```python
from build123d import *

# Parameters (mm, degrees)
BODY_DEPTH               = 10
SKETCH2_R                = 7.25
SPRING_HOLE_DEPTH        = 10
SKETCH3_R                = 3.25
SHAFT_HOLE_DEPTH         = 51.249378106
FIXATION_HOLE_START      = -20
SKETCH4_R                = 2.75
FIXATION_HOLE_DEPTH      = 72.478150705
SKETCH6_W                = 6
SKETCH6_H                = 10.5
NUT_HOLE_DEPTH           = 20
SKETCH7_R                = 3.2
INSERTS_TOP_DEPTH        = 9.5
SKETCH8_R                = 4.5
M5_SCREW_PLACE_DEPTH     = 5
SKETCH9_R                = 6.2
LINEARBEARINGPLACE_DEPTH = 19
CHAMFER1_SIZE            = 1
CHAMFER2_SIZE            = 1


with BuildPart() as part:
    # Sketch1 → Body (new, symmetric)
    with BuildSketch(Plane(origin=(0, 0, 0), x_dir=(1, 0, 0), z_dir=(0, 1, 0))):
        Polygon((-45, 15), (45, 15), (45, -5), (45, -15), (25, -15), (25, 0), (-25, 0), (-25, -15), (-45, -15), (-45, -5), align=None)
    extrude(amount=BODY_DEPTH, both=True)

    # Sketch2 → Spring_Hole (cut)
    with BuildSketch(Plane.XY.offset(15)):
        with Locations((-35, 0)):
            Circle(SKETCH2_R)
    spring_hole = extrude(amount=-SPRING_HOLE_DEPTH, mode=Mode.SUBTRACT)

    # Sketch3 → Shaft_Hole (cut, symmetric)
    with BuildSketch(Plane.XY.offset(5)):
        with Locations((-35, 0)):
            Circle(SKETCH3_R)
    shaft_hole = extrude(amount=SHAFT_HOLE_DEPTH, both=True, mode=Mode.SUBTRACT)

    # Sketch4 → Fixation_Hole (cut, through all)
    with BuildSketch(Plane(origin=(0, 10, 0), x_dir=(1, 0, 0), z_dir=(0, 1, 0)).offset(FIXATION_HOLE_START)):
        with Locations(Location((-18, 7.5, 0), (0, 0, 270))):
            Circle(SKETCH4_R)
    fixation_hole = extrude(amount=FIXATION_HOLE_DEPTH, mode=Mode.SUBTRACT)

    # Sketch6 → Nut_Hole (cut)
    with BuildSketch(Plane.ZY.offset(45)):
        with Locations((-7.5, 0)):
            Rectangle(SKETCH6_W, SKETCH6_H)
    nut_hole = extrude(amount=-NUT_HOLE_DEPTH, mode=Mode.SUBTRACT)

    # Mirror1: Spring_Hole, Shaft_Hole, Fixation_Hole, Nut_Hole across plane
    add(spring_hole.mirror(Plane(origin=(0, 0, 0), x_dir=(0, 0, 1), z_dir=(1, 0, 0))), mode=Mode.SUBTRACT)
    add(shaft_hole.mirror(Plane(origin=(0, 0, 0), x_dir=(0, 0, 1), z_dir=(1, 0, 0))), mode=Mode.SUBTRACT)
    add(fixation_hole.mirror(Plane(origin=(0, 0, 0), x_dir=(0, 0, 1), z_dir=(1, 0, 0))), mode=Mode.SUBTRACT)
    add(nut_hole.mirror(Plane(origin=(0, 0, 0), x_dir=(0, 0, 1), z_dir=(1, 0, 0))), mode=Mode.SUBTRACT)

    # Sketch7 → Inserts_Top (cut)
    with BuildSketch(Plane(origin=(0, 0, -15), x_dir=(-1, 0, 0), z_dir=(0, 0, -1))):
        with Locations((-10, 0)):
            Circle(SKETCH7_R)
        with Locations(Location((10, 0, 0), (0, 0, 180))):
            Circle(SKETCH7_R)
    extrude(amount=-INSERTS_TOP_DEPTH, mode=Mode.SUBTRACT)

    # Sketch8 → M5_Screw_Place (cut)
    with BuildSketch(Plane.XZ.offset(10)):
        with Locations(Location((-18, -7.5, 0), (0, 0, 270))):
            Circle(SKETCH8_R)
        with Locations(Location((18, -7.5, 0), (0, 0, 270))):
            Circle(SKETCH8_R)
    extrude(amount=-M5_SCREW_PLACE_DEPTH, mode=Mode.SUBTRACT)

    # Sketch9 → LinearBearingPlace (cut)
    with BuildSketch(Plane(origin=(0, 0, -15), x_dir=(-1, 0, 0), z_dir=(0, 0, -1))):
        with Locations((-35, 0)):
            Circle(SKETCH9_R)
    linearbearingplace = extrude(amount=-LINEARBEARINGPLACE_DEPTH, mode=Mode.SUBTRACT)

    # Mirror2: LinearBearingPlace across plane
    add(linearbearingplace.mirror(Plane(origin=(0, 0, 0), x_dir=(0, 0, 1), z_dir=(1, 0, 0))), mode=Mode.SUBTRACT)

    # Chamfer1
    chamfer1_edges = [part.edges().sort_by_distance(p)[0] for p in [
        (0, -10, 0),
        (-25, -10, 7.5),
        (-35, -10, 15),
        (-45, -10, 0),
        (45, -10, 0),
        (45, 10, 0),
        (35, -10, 15),
        (25, -10, 7.5),
        (-25, 0, 15),
        (-45, 0, 15),
        (45, 0, 15),
        (25, 0, 15),
        (-45, 10, 0),
        (-35, 10, 15),
        (-25, 10, 7.5),
        (0, 10, 0),
        (25, 10, 7.5),
        (35, 10, 15),
    ]]
    chamfer(chamfer1_edges, length=CHAMFER1_SIZE)

    # Chamfer2
    chamfer2_edges = [part.edges().sort_by_distance(p)[0] for p in [
        (-45, 0, -4.5),
        (-45, 5.25, -7.5),
        (-45, 0, -10.5),
        (-45, -5.25, -7.5),
        (45, 0, -4.5),
        (45, 5.25, -7.5),
        (45, 0, -10.5),
        (45, -5.25, -7.5),
    ]]
    chamfer(chamfer2_edges, length=CHAMFER2_SIZE)


solid = part.part
```
Here's how the part is built. I have some questions about the finished solid (model axes, mm). A direction names the side the tool comes from. Coordinates: 2 decimals unless noted, no trailing zeros. Write each loop counter-clockwise with the first axis right and the second up, starting at its lowest first coordinate (ties: lowest second). Pieces come first, ordered by that corner, then holes. Notation, with made-up numbers: (71, -31.75) -> (83, -31.75) arc R17 ccw to (83, -8.75) -> close; hole circle Ø9 at (63, 55). An arc over 180 degrees is marked (long way). Use a Markdown table: item, result. Add a question column.
(1) I'm going to push flat-ended pins straight in: P1, Ø3, axis at y = -2, z = -6.5, coming from the -X side; P2, Ø3, axis at y = 0.5, z = -8, coming from the +X side; P3, Ø2.5, axis at x = 17, z = -8, coming from the -Y side; P4, Ø11, axis at x = 35, y = 0, coming from the +Z side. Where does each tip first touch, or does it pass through?
(2) If we section it at D-D, the plane x = 10: Write out the boundary of the cut face in (y, z), and give its area (3 significant figures).
(3) If we section it at A-A, the plane x = -35: Write out the boundary of the cut face in (y, z), and give its area (3 significant figures).
(4) For faces 1 (the flat face through (-42, 0, -10.5)), 2 (the cylindrical face through (36.344, -6.053, -5.633)), 3 (the flat face through (42, 0, -4.5)), which set-ups out of +Z, -Z, +X, -X, +Y, -Y let a thin tool reach every point of the face, with its end or its side?
(5) We'd pull the mould along Y, two halves only. Please class faces 4 (the flat face through (-25, 0, 7)), 5 (the flat face through (41, -5.25, -8)): +Y half, -Y half, draft (parallel to the pull), parting line (faces both ways), or undercut.
(6) Please list where these lines run through material, in increasing order: line 1 (X direction, y = -6.65, z = -7.5); line 2 (Y direction, x = -35, z = -2.25); line 3 (X direction, y = -9, z = 1).
(7) If we section it at B-B, the plane z = -7.5: State how many separate pieces and enclosed holes the cut face has, and give its area (3 significant figures).
Outcome:
| question | item | result |
|---|---|---|
| 1 | P1 | stops at x = -25 |
| 1 | P2 | stops at x = 25 |
| 1 | P3 | passes through |
| 1 | P4 | stops at z = 5 |
| 2 | outline | (-10, -15) -> (-3.2, -15) -> (-3.2, -5.5) -> (3.2, -5.5) -> (3.2, -15) -> (10, -15) -> (10, -1) -> (9, 0) -> (-9, 0) -> (-10, -1) -> close |
| 2 | area | 238 mm^2 |
| 3 | outline | (-10, -15) -> (-6.2, -15) -> (-6.2, 4) -> (-3.25, 4) -> (-3.25, 5) -> (-7.25, 5) -> (-7.25, 15) -> (-9, 15) -> (-10, 14) -> close; (3.25, 4) -> (6.2, 4) -> (6.2, -15) -> (10, -15) -> (10, 14) -> (9, 15) -> (7.25, 15) -> (7.25, 5) -> (3.25, 5) -> close |
| 3 | area | 212 mm^2 |
| 4 | face 1 | -X |
| 4 | face 2 | -Z |
| 4 | face 3 | +X |
| 5 | face 4 | draft |
| 5 | face 5 | undercut |
| 6 | line 1 | x = -45 to -22.5, -13.5 to 13.5, 22.5 to 45 |
| 6 | line 2 | y = -10 to -6.2, 6.2 to 10 |
| 6 | line 3 | x = -45 to -25, 25 to 45 |
| 7 | separate pieces | 3 |
| 7 | enclosed holes | 2 |
| 7 | area | 1,040 mm^2 |
